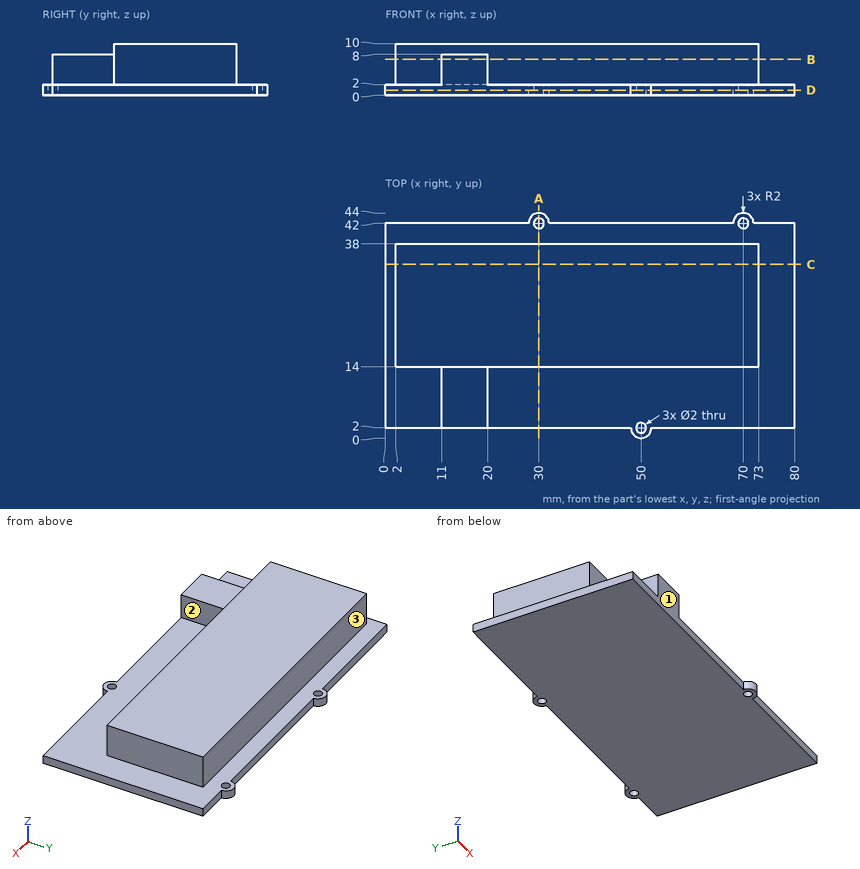
Answer from the drawing. Dimensions are ordinates in mm from the lowest x, y and z of the part. A direction names the side the tool comes from. Round coordinates to 2 decimals unless told otherwise and drop trailing zeros. Loops run counter-clockwise (first coordinate to the right, second up) from the corner with the lowest first, then second, coordinate; pieces in that order, holes last.
Q1. Which of the six approach directions +Z, -Z, +X, -X, +Y, -Y give full straight-line access (tool end or side, diameter ignored) to the marked faces 1, 2 and 3?
Q2. Section D-D on z = 1 is taken. Write down the section's boundary in (x, y), and give its area (3 significant figures).
Q3. Each of these flat-tipped pins is pushed along its axis until it touches: pin 1 (3 mm diameter, centred on x = 36.5, y = 10, fed in from +Z); pin 2 (4 mm diameter, centred on x = 15, z = 5.5, fed in from -Y); pin 3 (1 mm diameter, centred on x = 33, z = 7, fed in from -Y); pin 4 (1.6 mm diameter, centred on x = 70, y = 42, fed in from -Z) (3 decimals). Where does it stop, or does it pass through?
Q4. Consider probe 1 along Y at (x, z) = (70, 0.4); probe 2 along Y at (x, z) = (50, 0.5); probe 3 along X at (y, z) = (33, 7.25). Determine where each line is inside the solid, lowest interval first.
Q5. Section B-B on z = 7 is taken. Write down the section's boundary in (x, y).
Q6. Section A-A on x = 30 is taken. Write down the section's boundary in (y, z).
Q7. Section C-C on y = 34 is taken. Write down the section's boundary in (x, z), and give its area (3 significant figures).
Output:
1. face 1: +Z, -Z, -X, -Y
1. face 2: +Z, +X, -Y
1. face 3: +Z, +X, -X, +Y
2. outline: (0, 2) - (48, 2) arc R2 ccw to (52, 2) - (80, 2) - (80, 42) - (72, 42) arc R2 ccw to (68, 42) - (32, 42) arc R2 ccw to (28, 42) - (0, 42) - close; hole circle Ø2 at (30, 42); hole circle Ø2 at (50, 2); hole circle Ø2 at (70, 42)
2. area: 3,210 mm2
3. pin 1: stops at z = 2
3. pin 2: stops at y = 2
3. pin 3: stops at y = 14
3. pin 4: passes through
4. probe 1: y = 2 to 41, 43 to 44
4. probe 2: y = 0 to 1, 3 to 42
4. probe 3: x = 2 to 73
5. outline: (2, 14) - (11, 14) - (11, 2) - (20, 2) - (20, 14) - (73, 14) - (73, 38) - (2, 38) - close
6. outline: (2, 0) - (41, 0) - (41, 2) - (38, 2) - (38, 10) - (14, 10) - (14, 2) - (2, 2) - close; (43, 0) - (44, 0) - (44, 2) - (43, 2) - close
7. outline: (0, 0) - (80, 0) - (80, 2) - (73, 2) - (73, 10) - (2, 10) - (2, 2) - (0, 2) - close
7. area: 728 mm2
